Autodesk Inventor part; units mm, degrees
ref_plane "YZ Plane" through (0, 0, 0) normal (1, 0, 0) x (0, 1, 0)
ref_plane "XZ Plane" through (0, 0, 0) normal (0, 1, 0) x (-1, 0, 0)
ref_plane "XY Plane" through (0, 0, 0) normal (0, 0, 1) x (1, 0, 0)
sketch "Sketch1" plane through (0, 0, 0) normal (0, 1, 0) x (-1, 0, 0)
  point P0 (0, 0)
sketch "Sketch2" plane through (0, 0, 0) normal (0, 1, 0) x (-1, 0, 0)
  circle A0 centre (0, 0) radius 15.15
  circle A1 centre (0, 0) radius 17.65
  circle A2 centre (0, 0) radius 22.55
  circle A3 centre (0, 0) radius 20.05
  dimension "d0" = 30.3
  dimension "d1" = 2.5
  dimension "d2" = 45.1
  dimension "d3" = 2.5
extrude "Extrusion1" add sketch "Sketch2" along normal blind 9.5 contours A1 | A2 | A3
sketch "Sketch3" plane through (0, 0, 0) normal (0, -1, 0) x (1, 0, 0)
  circle A0 centre (0, 0) radius 15.15
  circle A1 centre (0, 0) radius 9
  dimension "d8" = 18
extrude "Extrusion2" add sketch "Sketch3" against normal blind 1.5
chamfer "Chamfer1" distance 0.5 angle 45 3 edges at (22.55, 0, 0) (15.15, 9.5, 0) (22.55, 9.5, 0)
properties part number "Bearing Spacer"
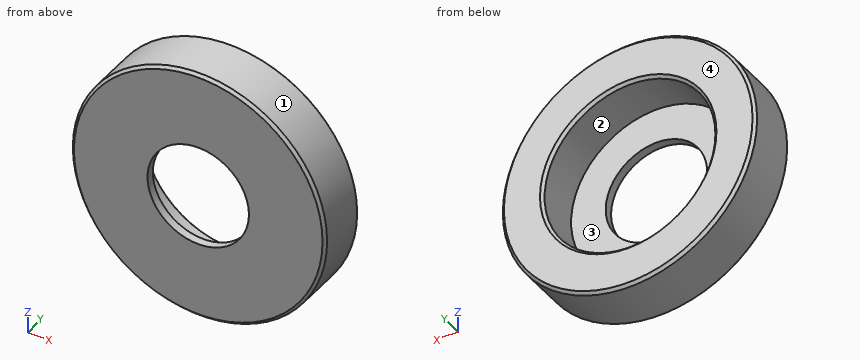
For this review, take the finished solid that the model builds, in its own axes (mm). Face numbers are marked on the shaded views. Round coordinates to 2 decimals unless told otherwise and drop trailing zeros. Order: outer loops, then holes, each group sorted by start corner. A loop starts at its lowest first (then second) coordinate and runs counter-clockwise, first axis right, second up. Notation, with made-up numbers: (87.25, 47) -> (116.25, 47) arc R22 cw to (116.25, 76) -> close; hole circle Ø7 at (56, 38.5). An arc over 180 degrees is marked (long way). Use a Markdown table: item, result.
Item 1: Take a section at A-A (x = 0). State the section outline as (y, z) points, plus the area to 3 significant figures.
Resolved:
| item | result |
|---|---|
| outline | (0, -22.05) -> (0.5, -22.55) -> (9, -22.55) -> (9.5, -22.05) -> (9.5, -15.65) -> (9, -15.15) -> (1.5, -15.15) -> (1.5, -9) -> (0, -9) -> close; (0, 9) -> (1.5, 9) -> (1.5, 15.15) -> (9, 15.15) -> (9.5, 15.65) -> (9.5, 22.05) -> (9, 22.55) -> (0.5, 22.55) -> (0, 22.05) -> close |
| area | 158 mm² |
Item 2: For pin 1 (1.5 mm diameter, centred on y = 8.5, z = -17, fed in from +X); pin 2 (1.5 mm diameter, centred on x = -2, y = 5.5, fed in from +Z); pin 3 (15 mm diameter, centred on x = -5.5, z = 0.5, fed in from +Y), all flat-tipped, find the tip position at first contact; note any pin that passes through.
Resolved:
| item | result |
|---|---|
| pin 1 | stops at x = 15.63 |
| pin 2 | stops at z = 22.52 |
| pin 3 | stops at y = 1.5 |
Item 3: Draft analysis for pull direction Z (two halves, no side actions). For the marked faces 1, 2, 3 and 4, state which applies: +Z half, -Z half, draft (parallel to the pull), parting line (faces both ways), or undercut.
Resolved:
| item | result |
|---|---|
| face 1 | parting line |
| face 2 | undercut |
| face 3 | undercut |
| face 4 | draft |
Item 4: Take a section at C-C (y = 5.5). State the section outline as (x, z) points.
Resolved:
| item | result |
|---|---|
| outline | circle Ø45.1 at (0, 0); hole circle Ø30.3 at (0, 0) |
Item 5: Take a section at B-B (z = 0). State the section outline as (x, y) points.
Resolved:
| item | result |
|---|---|
| outline | (-22.55, 0.5) -> (-22.05, 0) -> (-9, 0) -> (-9, 1.5) -> (-15.15, 1.5) -> (-15.15, 9) -> (-15.65, 9.5) -> (-22.05, 9.5) -> (-22.55, 9) -> close; (9, 0) -> (22.05, 0) -> (22.55, 0.5) -> (22.55, 9) -> (22.05, 9.5) -> (15.65, 9.5) -> (15.15, 9) -> (15.15, 1.5) -> (9, 1.5) -> close |
Item 6: For line 1 along Z through (x, y) = (0, 0.5); line 2 along Z through (x, y) = (0, 3); line 3 along Y through (x, z) = (-14, -5), list the stretches that pass through material, from the lowest coordinate up. Write a range as [from, to].
Resolved:
| item | result |
|---|---|
| line 1 | z = [-22.55, -9], [9, 22.55] |
| line 2 | z = [-22.55, -15.15], [15.15, 22.55] |
| line 3 | y = [0, 1.5] |
